For this review, take the finished solid that the model builds, in its own axes (mm). A direction names the side the tool comes from. Round coordinates to 2 decimals unless told otherwise and drop trailing zeros. Order: outer loops, then holes, each group sorted by start corner. A loop starts at its lowest first (then second) coordinate and runs counter-clockwise, first axis right, second up. Notation, with made-up numbers: (32.5, -40) - (63.5, -40) arc R32 cw to (63.5, -7) - close; hole circle Ø4 at (52.5, 36). An arc over 180 degrees is marked (long way). One line per item, written item: value.
```python
from build123d import *

# Parameters (mm, degrees)
CUT_EXTRUDE2_DEPTH  = 76.605010416
CUT_EXTRUDE3_DEPTH  = 76.605010416
BOSS_EXTRUDE1_START = 3.81
BOSS_EXTRUDE1_DEPTH = 3.81
SKETCH8_R           = 3.81
SKETCH8_R_2         = 1.397
BOSS_EXTRUDE2_DEPTH = 1.27


with BuildPart() as part:
    # Sketch1 → Revolve1 (revolve)
    with BuildSketch(Plane(origin=(0, 0, 0), x_dir=(1, 0, 0), z_dir=(0, 1, 0))):
        with BuildLine():
            Line((-53.34, 0), (-53.34, -0.635))
            ThreePointArc((-53.34, -0.635), (-51.435, -2.54), (-53.34, -4.445))
            Line((-53.34, -4.445), (-53.34, -5.08))
            Line((-53.34, -5.08), (0, -5.08))
            Line((0, -5.08), (0, 0))
            Line((0, 0), (-53.34, 0))
        make_face()
    revolve(axis=Axis((0, 0, 0), (0, 0, 1)))

    # Sketch3 → Cut-Extrude2 (cut, through all)
    with BuildSketch(Plane(origin=(0, 0, 0), x_dir=(-1, 0, 0), z_dir=(0, 0, -1))):
        with BuildLine():
            Line((2.794, 48.179053166), (2.794, 5.702285857))
            ThreePointArc((2.794, 5.702285857), (4.490128061, 4.490128061), (5.702285857, 2.794))
            Line((5.702285857, 2.794), (48.179053166, 2.794))
            ThreePointArc((48.179053166, 2.794), (34.12497326, 34.12497326), (2.794, 48.179053166))
        make_face()
        with BuildLine():
            Line((2.794, -5.702285857), (2.794, -48.179053166))
            ThreePointArc((2.794, -48.179053166), (34.12497326, -34.12497326), (48.179053166, -2.794))
            Line((48.179053166, -2.794), (5.702285857, -2.794))
            ThreePointArc((5.702285857, -2.794), (4.490128061, -4.490128061), (2.794, -5.702285857))
        make_face()
        with BuildLine():
            Line((-5.702285857, -2.794), (-48.179053166, -2.794))
            ThreePointArc((-48.179053166, -2.794), (-34.12497326, -34.12497326), (-2.794, -48.179053166))
            Line((-2.794, -48.179053166), (-2.794, -5.702285857))
            ThreePointArc((-2.794, -5.702285857), (-4.490128061, -4.490128061), (-5.702285857, -2.794))
        make_face()
        with BuildLine():
            Line((-2.794, 5.702285857), (-2.794, 48.179053166))
            ThreePointArc((-2.794, 48.179053166), (-34.12497326, 34.12497326), (-48.179053166, 2.794))
            Line((-48.179053166, 2.794), (-5.702285857, 2.794))
            ThreePointArc((-5.702285857, 2.794), (-4.490128061, 4.490128061), (-2.794, 5.702285857))
        make_face()
    extrude(amount=-CUT_EXTRUDE2_DEPTH, mode=Mode.SUBTRACT)

    # Sketch6 → Cut-Extrude3 (cut, through all)
    with BuildSketch(Plane(origin=(0, 0, 0), x_dir=(-1, 0, 0), z_dir=(0, 0, -1))):
        with BuildLine():
            Line((-2.159, 1.96747554), (-2.159, -1.96747554))
            ThreePointArc((-2.159, -1.96747554), (0, -2.921), (2.159, -1.96747554))
            Line((2.159, -1.96747554), (2.159, 1.96747554))
            ThreePointArc((2.159, 1.96747554), (0, 2.921), (-2.159, 1.96747554))
        make_face()
    extrude(amount=-CUT_EXTRUDE3_DEPTH, mode=Mode.SUBTRACT)

    # Sketch7 → Boss-Extrude1 (add)
    with BuildSketch(Plane(origin=(0, 0, 0), x_dir=(-1, 0, 0), z_dir=(0, 0, -1)).offset(BOSS_EXTRUDE1_START)):
        with BuildLine():
            Line((3.429, -2.409655577), (3.429, 2.409655577))
            ThreePointArc((3.429, 2.409655577), (0, 4.191), (-3.429, 2.409655577))
            Line((-3.429, 2.409655577), (-3.429, -2.409655577))
            ThreePointArc((-3.429, -2.409655577), (0, -4.191), (3.429, -2.409655577))
        make_face()
        with BuildLine():
            Line((2.159, -1.96747554), (2.159, 1.96747554))
            ThreePointArc((2.159, 1.96747554), (0, 2.921), (-2.159, 1.96747554))
            Line((-2.159, 1.96747554), (-2.159, -1.96747554))
            ThreePointArc((-2.159, -1.96747554), (0, -2.921), (2.159, -1.96747554))
        make_face(mode=Mode.SUBTRACT)
    extrude(amount=-BOSS_EXTRUDE1_DEPTH)

    # Sketch8 → Boss-Extrude2 (add)
    with BuildSketch(Plane.XY.offset(5.08)):
        Circle(SKETCH8_R)
        Circle(SKETCH8_R_2, mode=Mode.SUBTRACT)
    extrude(amount=-BOSS_EXTRUDE2_DEPTH)


solid = part.part
```
Item 1: The part is to be moulded in two halves that separate along X. For faces 1 (the cylindrical face through (0.06, -4.19, -1.93)), 2 (the flat face through (2.33, 0.06, -3.81)), 3 (the cylindrical face through (-34.471, 33.776, 2.504)), say which applies: +X half, -X half, draft (parallel to the pull), parting line (faces both ways), or undercut.
Returned:
face 1: parting line
face 2: draft
face 3: undercut
Item 2: For P1, Ø1.3, axis at x = -0.5, y = -1.5, coming from the -Z side; P2, Ø1.5, axis at y = -29, z = 2.5, coming from the +X side; P3, Ø2, axis at y = -0.5, z = -1.5, coming from the +X side, all flat-tipped, find the tip position at first contact; note any pin that passes through.
Returned:
P1: z = 3.81
P2: x = 42.98
P3: x = 3.43
Item 3: Take a section at B-B (x = 0). Write out the cut boundary in (y, z) (3 decimals), plus the area to 3 significant figures.
Returned:
outline: (-53.34, 0) - (-4.191, 0) - (-4.191, -3.81) - (-2.921, -3.81) - (-2.921, 3.81) - (-1.397, 3.81) - (-1.397, 5.08) - (-53.34, 5.08) - (-53.34, 4.445) arc R1.905 cw to (-53.34, 0.635) - close; (1.397, 3.81) - (2.921, 3.81) - (2.921, -3.81) - (4.191, -3.81) - (4.191, 0) - (53.34, 0) - (53.34, 0.635) arc R1.905 cw to (53.34, 4.445) - (53.34, 5.08) - (1.397, 5.08) - close
area: 514 mm^2
Item 4: Machinability: for faces 4 (the cylindrical face through (-0.06, 4.19, -1.93)), 5 (the cylindrical face through (-0.03, 2.92, -0.05)), 6 (the flat face through (-3.429, 0, -2)), 7 (the cylindrical face through (-4.51, -4.47, 2.5)), which of the approach directions +Z, -Z, +X, -X, +Y, -Y give a long, thin tool a straight path to every point of the face, cutting with its end or side? Answer none if there is none.
Returned:
face 4: -Z, +Y
face 5: -Z
face 6: -Z, -X, +Y, -Y
face 7: +Z, -Z
Item 5: Take a section at A-A (y = 0). Write out the cut boundary in (x, z) (3 decimals), plus the area to 3 significant figures.
Returned:
outline: (-53.34, 0) - (-3.429, 0) - (-3.429, -3.81) - (-2.159, -3.81) - (-2.159, 3.81) - (-1.397, 3.81) - (-1.397, 5.08) - (-53.34, 5.08) - (-53.34, 4.445) arc R1.905 cw to (-53.34, 0.635) - close; (1.397, 3.81) - (2.159, 3.81) - (2.159, -3.81) - (3.429, -3.81) - (3.429, 0) - (53.34, 0) - (53.34, 0.635) arc R1.905 cw to (53.34, 4.445) - (53.34, 5.08) - (1.397, 5.08) - close
area: 520 mm^2
Item 6: Take a section at C-C (y = 12). Count the separate pieces of the cut face and the enclosed holes in it, plus the area to 3 significant figures.
Returned:
separate pieces: 3
enclosed holes: 0
area: 69.8 mm^2
Item 7: Wall thickness on line 1 (X direction, y = 13, z = 1.75); line 2 (Y direction, x = 0, z = 4.5); line 3 (X direction, y = -6.5, z = 2.5): over which ranges is each line inside the solid? List them lowest first.
Returned:
line 1: -49.94 to -46.48, -2.79 to 2.79, 46.48 to 49.94
line 2: -53.34 to -1.4, 1.4 to 53.34
line 3: -51.02 to -47.82, -2.79 to 2.79, 47.82 to 51.02
